```python
from build123d import *

# Parameters (mm, degrees)
SKETCH_6_R             = 2
CUT_EXTRUDE_1_DEPTH    = 0.2
SKETCH_6_2_R           = 2
CUT_EXTRUDE_2_DEPTH    = 5
HOLE_WIZARD_M3_1_D     = 2.5
HOLE_WIZARD_M3_1_DEPTH = 5.5
HOLE_WIZARD_M3_1_TIP   = 0.751075774
SKETCH_10_R            = 10.599002553
CUT_EXTRUDE_3_DEPTH    = 10
SKETCH_11_R            = 1.5
EXTRUDE_1_DEPTH        = 5
FILLET_1_R             = 0.2
CHAMFER_1_SIZE         = 0.15


with BuildPart() as part:
    # 草图1 → 旋转1 (revolve)
    with BuildSketch(Plane.XY):
        with BuildLine():
            Line((0, 5), (0, -5))
            ThreePointArc((0, -5), (5, 0), (0, 5))
        make_face()
    revolve(axis=Axis((0, 5, 0), (0, -1, 0)))

    # 草图6 → 切除-拉伸1 (cut)
    with BuildSketch(Plane(origin=(-0.316240488, -4.7, 0), x_dir=(0.9977440075226778, -0.06713341532044086, 0), z_dir=(-0.06713341532044086, -0.9977440075226779, 0))):
        Circle(SKETCH_6_R)
    extrude(amount=-CUT_EXTRUDE_1_DEPTH, mode=Mode.SUBTRACT)


with BuildPart() as cut_extrude_1_piece_1:
    # of the separate pieces the step leaves, piece 1, a body of its own (cut_extrude_1_pieces)
    add(part.part.solids().sort_by_distance((1.687844058, -4.706504269, 0))[0])

    # M3 螺纹孔1
    with Locations(Plane(origin=(-0.302813805, -4.500451198, 0), x_dir=(-0.997744007523, 0.06713341532, 0), z_dir=(-0.06713341532, -0.997744007523, 0))):
        with Locations((0, 0)):
            Hole(HOLE_WIZARD_M3_1_D / 2, depth=HOLE_WIZARD_M3_1_DEPTH)
            with Locations((0, 0, -(HOLE_WIZARD_M3_1_DEPTH + HOLE_WIZARD_M3_1_TIP / 2))):  # 118° drill point
                Cone(0, HOLE_WIZARD_M3_1_D / 2, HOLE_WIZARD_M3_1_TIP, mode=Mode.SUBTRACT)

    # 草图10 → 切除-拉伸3 (cut)
    with BuildSketch(Plane(origin=(3.8, 0, 0), x_dir=(0, 0, -1), z_dir=(1, 0, 0))):
        Circle(SKETCH_10_R)
    extrude(amount=CUT_EXTRUDE_3_DEPTH, mode=Mode.SUBTRACT)

    # 草图11 → 凸台-拉伸1 (add)
    with BuildSketch(Plane(origin=(3.8, 0, 0), x_dir=(0, 0, -1), z_dir=(1, 0, 0))):
        Circle(SKETCH_11_R)
    extrude(amount=EXTRUDE_1_DEPTH)

    # 圆角1
    fillet_1_edges = [cut_extrude_1_piece_1.edges().sort_by_distance(p)[0] for p in [
        (3.8, 0, -3.249615362),
    ]]
    fillet(fillet_1_edges, radius=FILLET_1_R)

    # 倒角1
    chamfer_1_edges = [cut_extrude_1_piece_1.edges().sort_by_distance(p)[0] for p in [
        (8.8, 0, 1.5),
    ]]
    chamfer(chamfer_1_edges, length=CHAMFER_1_SIZE)


with BuildPart() as cut_extrude_1_piece_2:
    # of the separate pieces the step leaves, piece 2, a body of its own (cut_extrude_1_pieces)
    add(part.part.solids().sort_by_distance((0, -5, 0))[0])

    # 草图6<2> → 切除-拉伸2 (cut)
    with BuildSketch(Plane(origin=(-0.316240488, -4.7, 0), x_dir=(0.9977440075226778, -0.06713341532044086, 0), z_dir=(-0.06713341532044086, -0.9977440075226779, 0))):
        Circle(SKETCH_6_2_R)
    extrude(amount=CUT_EXTRUDE_2_DEPTH, mode=Mode.SUBTRACT)


solid = cut_extrude_1_piece_1.part
```
The listing builds one solid part. Answer for the finished solid, in the listing's coordinates (mm). Give positions to 0.01 mm unless a question says otherwise; leave off trailing zeros. Order: outer loops, then holes, each group sorted by start corner. A loop starts at its lowest first (then second) coordinate and runs counter-clockwise, first axis right, second up. Notation, with made-up numbers: M -27,-4 L 20,-4 A4 cw 20,0 Z; hole C 74,-33.75 d10. An arc over 180 degrees is marked long. Put each result on its own line as item: value. Start each with the question number.
Item 1: Flat-ended cylindrical pins translate along their axes: P1, Ø3, axis at y = -3, z = 3, coming from the -X side; P2, Ø1, axis at x = 7, z = -1, coming from the -Y side; P3, Ø5, axis at x = 2.5, z = 3, coming from the +Y side. Find the tip coordinate at first contact, or state that the pin passes through.
Item 2: For a pull along Y with two mould halves and no side action, classify faces 1 (the face through (6.19, 0.07, 1.5)), 2 (the face through (-0.39, -1.7, 1.22)), 3 (the face through (8.8, 0, 0)) as +Y half, -Y half, draft (parallel to the pull), parting line (faces both ways), or undercut.
Item 3: The part is cut by section B-B, the plane x = 7.5. Determine the outline of the cut face in (y, z).
Item 4: Find the intervals of material crossed by line 1 along Z through (x, y) = (-0.75, -3); line 2 along Z through (x, y) = (-0.75, -2.25); line 3 along X through (y, z) = (-2.25, 0.5), in increasing order.
Item 5: The part is cut by section A-A, the plane z = 4. Determine the outline of the cut face in (x, y).
Answer key:
1. P1: stops at x = -4.18
1. P2: stops at y = -1.41
1. P3: stops at y = 4.8
2. face 1: parting line
2. face 2: undercut
2. face 3: draft
3. outline: C 0,0 d3
4. line 1: z = -3.93 to -1.12, 1.12 to 3.93
4. line 2: z = -4.4 to -1.1, 1.1 to 4.4
4. line 3: x = -4.44 to -1.3, 1 to 3.8
5. outline: C 0,0 d6
